from build123d import *

# Parameters (mm, degrees)
BOSS_EXTRU_1_DEPTH      = 6
ESQUISSE2_R             = 10
ESQUISSE2_R_2           = 2
ESQUISSE2_R_3           = 1.4
ESQUISSE2_R_4           = 1.5
ESQUISSE2_W             = 8
ESQUISSE2_H             = 55
ESQUISSE2_W_2           = 44
ESQUISSE2_W_3           = 110
ESQUISSE2_H_2           = 60
ENL_V_MAT_EXTRU_1_DEPTH = 6
ESQUISSE3_W             = 6
ESQUISSE3_H             = 10
ESQUISSE3_W_2           = 15
ESQUISSE3_H_2           = 6
ENL_V_MAT_EXTRU_2_DEPTH = 6
ESQUISSE4_R             = 1.5
ENL_V_MAT_EXTRU_3_DEPTH = 6
ESQUISSE5_W             = 10
ESQUISSE5_H             = 6
ENL_V_MAT_EXTRU_4_DEPTH = 6
ESQUISSE6_R             = 1.65
ESQUISSE6_R_2           = 2
ENL_V_MAT_EXTRU_5_DEPTH = 6
ESQUISSE8_R             = 1.5
ESQUISSE8_W             = 6
ESQUISSE8_H             = 20
ENL_V_MAT_EXTRU_8_DEPTH = 6


with BuildPart() as part:
    # Esquisse1 → Boss.-Extru.1 (new body)
    with BuildSketch(Plane.XY):
        Polygon((-165, 96.73), (165, 96.73), (165, -18.27), (123, -109.022410436), (-123, -109.022410436), (-165, -18.27), align=None)
    extrude(amount=BOSS_EXTRU_1_DEPTH)

    # Esquisse2 → Enlèv. mat.-Extru.1 (cut)
    with BuildSketch(Plane.XY.offset(6)):
        with Locations((140, 76.73)):
            Circle(ESQUISSE2_R)
        with Locations((108, -89.022410436)):
            Circle(ESQUISSE2_R)
        with Locations(Location((-140, 76.73, 0), (0, 0, 180))):
            Circle(ESQUISSE2_R)
        with Locations(Location((-108, -89.022410436, 0), (0, 0, 180))):
            Circle(ESQUISSE2_R)
        with Locations((161, -16.022410436)):
            Circle(ESQUISSE2_R_2)
        with Locations((119, -105.022410436)):
            Circle(ESQUISSE2_R_2)
        with Locations((161, 92.73)):
            Circle(ESQUISSE2_R_2)
        with Locations(Location((-161, 92.73, 0), (0, 0, 180))):
            Circle(ESQUISSE2_R_2)
        with Locations(Location((-161, -16.022410436, 0), (0, 0, 180))):
            Circle(ESQUISSE2_R_2)
        with Locations(Location((-119, -105.022410436, 0), (0, 0, 180))):
            Circle(ESQUISSE2_R_2)
        with Locations((125.27, 76.73)):
            Circle(ESQUISSE2_R_3)
        with Locations((110.27, 76.73)):
            Circle(ESQUISSE2_R_3)
        with Locations((114.7893454, -75.950391119)):
            Circle(ESQUISSE2_R_4)
        with Locations((121.703139086, -62.638762485)):
            Circle(ESQUISSE2_R_4)
        with Locations(Location((-110.27, 76.73, 0), (0, 0, 180))):
            Circle(ESQUISSE2_R_3)
        with Locations(Location((-125.27, 76.73, 0), (0, 0, 180))):
            Circle(ESQUISSE2_R_3)
        with Locations(Location((-121.703139086, -62.638762485, 0), (0, 0, 180))):
            Circle(ESQUISSE2_R_4)
        with Locations(Location((-114.7893454, -75.950391119, 0), (0, 0, 180))):
            Circle(ESQUISSE2_R_4)
        with Locations((-154, 38.477589564)):
            Rectangle(ESQUISSE2_W, ESQUISSE2_H)
        with Locations((-108, 38.477589564)):
            Rectangle(ESQUISSE2_W_2, ESQUISSE2_H)
        with Locations((108, 38.477589564)):
            Rectangle(ESQUISSE2_W_2, ESQUISSE2_H)
        with Locations((154, 38.477589564)):
            Rectangle(ESQUISSE2_W, ESQUISSE2_H)
        with Locations((0, -79.022410436)):
            Rectangle(ESQUISSE2_W_3, ESQUISSE2_H_2)
    extrude(amount=-ENL_V_MAT_EXTRU_1_DEPTH, mode=Mode.SUBTRACT)

    # Esquisse3 → Enlèv. mat.-Extru.2 (cut)
    with BuildSketch(Plane(origin=(0, 0, 0), x_dir=(-1, 0, 0), z_dir=(0, 0, -1))):
        with Locations((162, 1.73)):
            Rectangle(ESQUISSE3_W, ESQUISSE3_H)
        with Locations((162, 83.852589564)):
            Rectangle(ESQUISSE3_W, ESQUISSE3_H)
        with Locations((-162, 83.852589564)):
            Rectangle(ESQUISSE3_W, ESQUISSE3_H)
        with Locations((-162, 1.73)):
            Rectangle(ESQUISSE3_W, ESQUISSE3_H)
        with Locations((107.5, 93.73)):
            Rectangle(ESQUISSE3_W_2, ESQUISSE3_H_2)
        with Locations((-42.5, 93.73)):
            Rectangle(ESQUISSE3_W_2, ESQUISSE3_H_2)
        with Locations((42.5, 93.73)):
            Rectangle(ESQUISSE3_W_2, ESQUISSE3_H_2)
        with Locations((-107.5, 93.73)):
            Rectangle(ESQUISSE3_W_2, ESQUISSE3_H_2)
    extrude(amount=-ENL_V_MAT_EXTRU_2_DEPTH, mode=Mode.SUBTRACT)

    # Esquisse4 → Enlèv. mat.-Extru.3 (cut)
    with BuildSketch(Plane(origin=(0, 0, 0), x_dir=(-1, 0, 0), z_dir=(0, 0, -1))):
        with Locations((162, -6.27)):
            Circle(ESQUISSE4_R)
        with Locations((162, 72.852589564)):
            Circle(ESQUISSE4_R)
        with Locations((0, 93.73)):
            Circle(ESQUISSE4_R)
        with Locations((150, 93.73)):
            Circle(ESQUISSE4_R)
        with Locations((125, 93.73)):
            Circle(ESQUISSE4_R)
        with Locations((90, 93.73)):
            Circle(ESQUISSE4_R)
        with Locations(Location((-25, 93.73, 0), (0, 0, 180))):
            Circle(ESQUISSE4_R)
        with Locations((60, 93.73)):
            Circle(ESQUISSE4_R)
        with Locations((25, 93.73)):
            Circle(ESQUISSE4_R)
        with Locations(Location((-60, 93.73, 0), (0, 0, 180))):
            Circle(ESQUISSE4_R)
        with Locations(Location((-90, 93.73, 0), (0, 0, 180))):
            Circle(ESQUISSE4_R)
        with Locations(Location((-125, 93.73, 0), (0, 0, 180))):
            Circle(ESQUISSE4_R)
        with Locations(Location((-150, 93.73, 0), (0, 0, 180))):
            Circle(ESQUISSE4_R)
        with Locations(Location((-162, 72.852589564, 0), (0, 0, 180))):
            Circle(ESQUISSE4_R)
        with Locations(Location((-162, -6.27, 0), (0, 0, 180))):
            Circle(ESQUISSE4_R)
    extrude(amount=-ENL_V_MAT_EXTRU_3_DEPTH, mode=Mode.SUBTRACT)

    # Esquisse5 → Enlèv. mat.-Extru.4 (cut)
    with BuildSketch(Plane(origin=(0, 0, 0), x_dir=(-1, 0, 0), z_dir=(0, 0, -1))):
        with Locations((80, -41.022410436)):
            Rectangle(ESQUISSE5_W, ESQUISSE5_H)
        with Locations((-80, -41.022410436)):
            Rectangle(ESQUISSE5_W, ESQUISSE5_H)
    extrude(amount=-ENL_V_MAT_EXTRU_4_DEPTH, mode=Mode.SUBTRACT)

    # Esquisse6 → Enlèv. mat.-Extru.5 (cut)
    with BuildSketch(Plane(origin=(0, 0, 0), x_dir=(-1, 0, 0), z_dir=(0, 0, -1))):
        with Locations((-140, 13.477589564)):
            Circle(ESQUISSE6_R)
        with Locations((-140, 63.477589564)):
            Circle(ESQUISSE6_R)
        with Locations(Location((140, 63.477589564, 0), (0, 0, 180))):
            Circle(ESQUISSE6_R)
        with Locations(Location((140, 13.477589564, 0), (0, 0, 180))):
            Circle(ESQUISSE6_R)
        with Locations((-78.5, 59.477589564)):
            Circle(ESQUISSE6_R_2)
        with Locations((-78.5, 17.477589564)):
            Circle(ESQUISSE6_R_2)
        with Locations((-60, 57.977589564)):
            Circle(ESQUISSE6_R_2)
        with Locations((-60, 18.977894939)):
            Circle(ESQUISSE6_R_2)
        with Locations((60, 18.977894939)):
            Circle(ESQUISSE6_R_2)
        with Locations((60, 57.977589564)):
            Circle(ESQUISSE6_R_2)
        with Locations((-50, 55.977589564)):
            Circle(ESQUISSE6_R_2)
        with Locations((50, 55.977589564)):
            Circle(ESQUISSE6_R_2)
        with Locations((50, 20.977589564)):
            Circle(ESQUISSE6_R_2)
        with Locations((-50, 20.977589564)):
            Circle(ESQUISSE6_R_2)
        with Locations(Location((78.5, 17.477589564, 0), (0, 0, 180))):
            Circle(ESQUISSE6_R_2)
        with Locations(Location((78.5, 59.477589564, 0), (0, 0, 180))):
            Circle(ESQUISSE6_R_2)
    extrude(amount=-ENL_V_MAT_EXTRU_5_DEPTH, mode=Mode.SUBTRACT)

    # Esquisse8 → Enlèv. mat.-Extru.8 (cut)
    with BuildSketch(Plane(origin=(0, 0, 0), x_dir=(-1, 0, 0), z_dir=(0, 0, -1))):
        with Locations((-36.5, -44.022410436)):
            Circle(ESQUISSE8_R)
        with Locations((-36.5, -14.022410436)):
            Circle(ESQUISSE8_R)
        with Locations(Location((36.5, -14.022410436, 0), (0, 0, 180))):
            Circle(ESQUISSE8_R)
        with Locations(Location((36.5, -44.022410436, 0), (0, 0, 180))):
            Circle(ESQUISSE8_R)
        with Locations((-36.5, -29.022410436)):
            Rectangle(ESQUISSE8_W, ESQUISSE8_H)
        with Locations((36.5, -29.022410436)):
            Rectangle(ESQUISSE8_W, ESQUISSE8_H)
    extrude(amount=-ENL_V_MAT_EXTRU_8_DEPTH, mode=Mode.SUBTRACT)


solid = part.part
Design review of the part built by this model. Coordinates are the model's own, in mm. A direction names the side the tool comes from. Give positions to 0.01 mm unless a question says otherwise; leave off trailing zeros. Order: outer loops, then holes, each group sorted by start corner. A loop starts at its lowest first (then second) coordinate and runs counter-clockwise, first axis right, second up. Notation, with made-up numbers: (-14, 31) - (43, 31) arc R22 cw to (43, 59) - close; hole circle Ø9 at (46.5, 49.25). An arc over 180 degrees is marked (long way). Write item = value, one per line. Start each with the question number.
Q1. We need section B-B on z = 4.7. State how many separate pieces and enclosed holes the cut face has, plus the area to 3 significant figures.
Q2. Mouldability with a two-part tool opening along X and no side actions: class faces 1 (the face through (43, 90.73, 3)), 2 (the face through (159, 2, 3)), 3 (the face through (-162, -3.27, 3)) as released by +X, released by -X, zero draft, split by the parting line, or undercut.
Q3. To check wall thickness, follow L1, parallel to X at y = -76, z = 1.75; L2, parallel to X at y = 48.5, z = 5.2; L3, parallel to Y at x = 78.5, z = 1.9. State the ranges of each line that lie inside material, in increasing order. Write a range as from..to.
Q4. Tool access review of faces 4 (the face through (-158, 38, 3)), 5 (the face through (165, -11, 3)), 6 (the face through (-162, 6.73, 3)), 7 (the face through (-75, 96.73, 3)), 8 (the face through (-42, 90.73, 3)): name each direction out of +Z, -Z, +X, -X, +Y, -Y from which nothing blocks a thin tool from reaching the whole face with its end or side.
Q5. We need section A-A on y = -57.5. State the section outline as (x, z) points.
Q6. Clearance check with flat-ended pins moving along their axes: pin 1 Ø3 at (x, z) = (152, 4.5) entering from -Y; pin 2 Ø1.8 at (y, z) = (82, 1.5) entering from -X; pin 3 Ø3 at (x, z) = (-50, 3) entering from -Y. State where each tip first meets the part, or that it passes through.
Working result:
q1.separate_pieces = 1
q1.enclosed_holes = 61
q1.area = 49,100 mm²
q2.face_1 = undercut
q2.face_2 = released by +X
q2.face_3 = zero draft
q3.L1 = -138.28..-116.29, -113.29..-55, 55..113.29, 116.29..138.28
q3.L2 = -165..-158, -150..-130, -86..86, 130..150, 158..165
q3.L3 = -109.02..-44.02, -38.02..15.48, 19.48..57.48, 61.48..96.73
q4.face_4 = +Z, -Z
q4.face_5 = +Z, -Z, +X, +Y, -Y
q4.face_6 = +Z, -Z, -X
q4.face_7 = +Z, -Z, +X, -X, +Y
q4.face_8 = +Z, -Z, +Y
q5.outline = (-146.84, 0) - (-55, 0) - (-55, 6) - (-146.84, 6) - close; (55, 0) - (146.84, 0) - (146.84, 6) - (55, 6) - close
q6.pin_1 = -49.6
q6.pin_2 = -159
q6.pin_3 = -49.02
